Here's how the part is built. I have some questions about the finished solid (model axes, mm). A direction names the side the tool comes from. Coordinates: 2 decimals unless noted, no trailing zeros. Write each loop counter-clockwise with the first axis right and the second up, starting at its lowest first coordinate (ties: lowest second). Pieces come first, ordered by that corner, then holes. Notation, with made-up numbers: M 82,33.25 L 98,33.25 A22 cw 98,70.25 Z; hole C 40.25,82 d9. An arc over 180 degrees is marked long. Use a Markdown table: item, result.
```python
from build123d import *

# Parameters (mm, degrees)
F1_DEPTH = 6.35


with BuildPart() as f1:
    # F0 (on Front) → F1 (new body)
    with BuildSketch(Plane.XZ):
        Polygon((-34.308497, 70.690155), (-35.627097, 72.361246), (-39.185513, 73.408395), (-45.085765, 74.37408), (-45.085765, 73.587187), (-45.627236, 70.428468), (-45.627236, 66.162765), (-44.614065, 63.659623), (-42.647313, 60.918093), (-39.607789, 57.407359), (-38.379731, 56.234379), (-52.432694, 31.958599), (-61.129313, 16.639169), (-68.144596, 3.424435), (-69.156672, 1.654225), (-69.156672, 0), (-66.961855, -4.073157), (-38.026095, -56.195294), (-39.102234, -57.228971), (-39.421171, -57.228971), (-43.712616, -61.858468), (-44.787329, -63.857928), (-45.862038, -66.007353), (-45.862038, -70.906028), (-45.462146, -73.80525), (-40.563464, -73.80525), (-37.146181, -72.502002), (-34.33761, -70.180252), (-34.33761, -69.318958), (-34.824431, -68.120629), (-35.535935, -67.221887), (-35.535935, -64.488217), (-35.198905, -64.488217), (-30.354133, -58.102311), (-29.960589, -57.83011), (-24.916569, -54.341327), (-17.60274, -50.432213), (-3.689651, -44.463456), (1.271262, -39.682169), (7.641939, -27.768502), (7.641939, -22.784742), (6.722947, -18.47255), (2.988683, -13.726575), (-1.459086, -10.381853), (-1.743743, -8.460417), (-0.960936, -8.460417), (-0.960936, -4.546382), (-0.539417, -4.546382), (-0.539417, -3.977067), (-0.539417, 4.104951), (-0.930821, 4.460773), (-0.930821, 8.268063), (-1.179896, 8.801795), (-1.179896, 10.829977), (1.248935, 12.272857), (5.584201, 17.022802), (7.657589, 24.788585), (7.318308, 28.822267), (4.647506, 34.791052), (-2.222107, 43.378066), (-19.41184, 51.835634), (-30.058911, 58.020536), (-28.905725, 61.441984), (-29.26437, 62.742077), (-30.878276, 64.946632), (-33.040687, 64.946632), (-34.285408, 63.728355), (-35.215292, 64.678423), (-35.483975, 67.398816), (-34.913026, 68.507127), (-34.308497, 70.018455), align=None)
        Polygon((-18.50041, -42.745914), (-34.824431, -53.119961), (-35.786382, -54.043956), (-39.810754, -47.711428), (-60.148131, -9.969187), (-66.390261, 0.486024), (-61.881507, 9.981615), (-36.214546, 54.166303), (-35.249628, 53.244662), (-28.627157, 49.176574), (-21.531653, 44.824664), (-16.328281, 41.702639), (-11.685591, 38.048264), (-7.752089, 34.472354), (-4.831761, 30.181259), (-3.937784, 26.247757), (-4.474171, 22.969838), (-5.72574, 20.585898), (-8.467271, 17.009988), (-11.089605, 14.804843), (-11.089605, 13.970464), (-9.57832, -3.704541), (-11.153418, -14.336454), (-6.371869, -18.836735), (-4.217299, -22.886988), (-4.217299, -24.904553), (-4.668344, -29.264662), (-6.472527, -32.472096), (-8.627522, -35.078138), (-12.486468, -38.736619), align=None, mode=Mode.SUBTRACT)
    extrude(amount=F1_DEPTH)


solid = f1.part
```
1. Will these pins go through, and if not, where does the flat tip stop? pin 1 Ø3 at (y, z) = (-2, 6) entering from +X; pin 2 Ø0.9 at (y, z) = (-2.5, -70) entering from +X; pin 3 Ø1.5 at (y, z) = (-1, -42) entering from +X.
Answers follow:
| item | result |
|---|---|
| pin 1 | stops at x = -0.93 |
| pin 2 | stops at x = -34.34 |
| pin 3 | stops at x = -0.36 |
2. I need wall thicknesses on probe 1 along Z at (x, y) = (-5.5, -4.5); probe 2 along X at (y, z) = (-2.5, 22.5); probe 3 along Z at (x, y) = (0, -2.25). Which ranges of each line are inside material? Lowest first, please.
Answers follow:
| item | result |
|---|---|
| probe 1 | z = -45.24 to -30.74, -20.48 to 21.02, 31.16 to 44.99 |
| probe 2 | x = -57.8 to -54.61, -4.72 to 7.05 |
| probe 3 | z = -40.91 to -11.48, 11.53 to 40.6 |
3. Suppose I cut it at B-B on z = -36.5. Write out the boundary of the cut face in (x, y).
Answers follow:
| item | result |
|---|---|
| outline | M -48.96,-6.35 L -45.85,-6.35 L -45.85,0 L -48.96,0 Z; M -10.13,-6.35 L 2.97,-6.35 L 2.97,0 L -10.13,0 Z |
4. Which directions (+Z, -Z, +X, -X, +Y, -Y) give clear straight access to the entire face, cutting with the end or side of a thin tool? Please do faces 4 (the face through (-29.49, -3.13, 59.71)), 5 (the face through (-56.72, -3.13, 24.41)), 6 (the face through (-5.56, -3.13, -30.85)).
Answers follow:
| item | result |
|---|---|
| face 4 | +X, +Y, -Y |
| face 5 | +Z, -X, +Y, -Y |
| face 6 | +Y, -Y |
5. Suppose I cut it at A-A on x = -55.5. Write out the boundary of the cut face in (y, z), and give its area (3 significant figures).
Answers follow:
| item | result |
|---|---|
| outline | M -6.35,-24.72 L 0,-24.72 L 0,-18.6 L -6.35,-18.6 Z; M -6.35,20.97 L 0,20.97 L 0,26.56 L -6.35,26.56 Z |
| area | 74.4 mm2 |
6. We'd pull the mould along Z, two halves only. Please class faces 1 (the face through (0.8, -3.13, -12.08)), 2 (the face through (-10.7, -3.13, 47.55)), 3 (the face through (-43, -3, -73.805)): +Z half, -Z half, draft (parallel to the pull), parting line (faces both ways), or undercut.
Answers follow:
| item | result |
|---|---|
| face 1 | undercut |
| face 2 | +Z half |
| face 3 | -Z half |
